Design review of the part built by this model. Coordinates are the model's own, in mm. A direction names the side the tool comes from. Round coordinates to 2 decimals unless told otherwise and drop trailing zeros. Loops run counter-clockwise (first coordinate to the right, second up) from the corner with the lowest first, then second, coordinate; pieces in that order, holes last. Notation, with made-up numbers: (-31.75, 20.25) - (9.25, 20.25) arc R37 ccw to (9.25, 58.25) - close; hole circle Ø10 at (53, -13). An arc over 180 degrees is marked (long way). Return JSON: item names as keys, results as strings. Group by question number.
from build123d import *

# Parameters (mm, degrees)
F0_W     = 279.4
F0_H     = 482.6
F1_DEPTH = 25.4
F3_DEPTH = 10


with BuildPart() as f1:
    # F0 (on Front) → F1 (new body)
    with BuildSketch(Plane.XZ):
        Rectangle(F0_W, F0_H)
        Polygon((-91.511846, 158.487543), (-91.511846, 182.334796), (98.073885, 182.334796), (98.073885, 158.487543), (98.073885, 134.640291), (-91.511846, 134.640291), align=None, mode=Mode.SUBTRACT)
    extrude(amount=F1_DEPTH)

    # F2 (on face) → F3 (join)
    with BuildSketch(Plane.XZ.offset(25.4)):
        with BuildLine():
            ThreePointArc((114.3, -28.713468), (96.339488, -21.273981), (88.9, -3.313468))
            Line((88.9, -3.313468), (88.9, -28.713468))
            Line((88.9, -28.713468), (114.3, -28.713468))
        make_face()
        with BuildLine():
            Line((139.7, -28.713468), (139.7, -3.313468))
            ThreePointArc((139.7, -3.313468), (132.260512, -21.273981), (114.3, -28.713468))
            Line((114.3, -28.713468), (139.7, -28.713468))
        make_face()
        with BuildLine():
            ThreePointArc((88.9, -3.313468), (96.339488, 14.647044), (114.3, 22.086532))
            Line((114.3, 22.086532), (88.9, 22.086532))
            Line((88.9, 22.086532), (88.9, -3.313468))
        make_face()
        with BuildLine():
            ThreePointArc((139.7, -3.313468), (132.260512, 14.647044), (114.3, 22.086532))
            ThreePointArc((114.3, 22.086532), (96.339488, 14.647044), (88.9, -3.313468))
            ThreePointArc((88.9, -3.313468), (96.339488, -21.273981), (114.3, -28.713468))
            ThreePointArc((114.3, -28.713468), (132.260512, -21.273981), (139.7, -3.313468))
        make_face()
        with BuildLine():
            Line((139.7, -3.313468), (139.7, 22.086532))
            Line((139.7, 22.086532), (114.3, 22.086532))
            ThreePointArc((114.3, 22.086532), (132.260512, 14.647044), (139.7, -3.313468))
        make_face()
    extrude(amount=F3_DEPTH)


solid = f1.part
Q1. Draft analysis for pull direction Z (two halves, no side actions). For faces 6 (the flat face through (-91.512, -13, 158)), 7 (the flat face through (-2, -13, 241.3)), 8 (the flat face through (114, -30, -28.713)), state which applies: pulls with the +Z half, pulls with the -Z half, needs draft (parallel to the pull), parting line crosses it, or undercut.
Q2. Add section C-C, the plane z = -151. State the section outline as (x, y) points.
Q3. Add section A-A, the plane x = -43.5. State the section outline as (y, z) points.
Q4. Add section B-B, the plane y = -5.5. State the section outline as (x, z) points.
Q5. For line 1 (Z direction, x = -83, y = -15.5); line 2 (X direction, y = -23.5, z = 178); line 3 (Y direction, x = 63.5, z = 62), list the stretches that pass through material, from the lowest coordinate up.
Q6. Insertion check: pin 1 Ø8 at (x, y) = (117.5, -31.5) entering from +Z; pin 2 Ø8 at (y, z) = (-30, -0.5) entering from -X; pin 3 Ø3 at (y, z) = (-27, 110.5) entering from +X; pin 4 Ø5 at (x, y) = (119, -31.5) entering from -Z. Each pin has a flat end and moves straight along its axis. Give the tip position at first contact, or say it passes through.
Q7. Add section D-D, the plane x = 106.5. State the section outline as (y, z) points.
Q8. Tool access review of faces 1 (the flat face through (115, -30, 22.087)), 2 (the flat face through (-2, -13, -241.3)), 3 (the flat face through (-139.7, -13, -3)), 4 (the flat face through (2, -13, 182.335)), 5 (the flat face through (88.9, -30, -3)): name each direction out of +Z, -Z, +X, -X, +Y, -Y from which nothing blocks a thin tool from reaching the whole face with its end or side.
Evaluation:
{
 "1": {"face 6": "undercut", "face 7": "pulls with the +Z half", "face 8": "pulls with the -Z half"},
 "2": {"outline": "(-139.7, -25.4) - (139.7, -25.4) - (139.7, 0) - (-139.7, 0) - close"},
 "3": {"outline": "(-25.4, -241.3) - (0, -241.3) - (0, 134.64) - (-25.4, 134.64) - close; (-25.4, 182.33) - (0, 182.33) - (0, 241.3) - (-25.4, 241.3) - close"},
 "4": {"outline": "(-139.7, -241.3) - (139.7, -241.3) - (139.7, 241.3) - (-139.7, 241.3) - close; hole (-91.51, 134.64) - (98.07, 134.64) - (98.07, 182.33) - (-91.51, 182.33) - close"},
 "5": {"line 1": "-241.3 to 134.64, 182.33 to 241.3", "line 2": "-139.7 to -91.51, 98.07 to 139.7", "line 3": "-25.4 to 0"},
 "6": {"pin 1": "z = 22.09", "pin 2": "x = 88.9", "pin 3": "through", "pin 4": "z = -28.71"},
 "7": {"outline": "(-35.4, -28.71) - (-25.4, -28.71) - (-25.4, -241.3) - (0, -241.3) - (0, 241.3) - (-25.4, 241.3) - (-25.4, 22.09) - (-35.4, 22.09) - close"},
 "8": {"face 1": "+Z, +X, -X, -Y", "face 2": "-Z, +X, -X, +Y, -Y", "face 3": "+Z, -Z, -X, +Y, -Y", "face 4": "+Y, -Y", "face 5": "+Z, -Z, -X, -Y"}
}
